```python
from build123d import *

# Parameters (mm, degrees)
BOSS_EXTRUDE1_DEPTH = 38.1
SHELL1_T            = -3.81
CUT_EXTRUDE1_DEPTH  = 3.81
BOSS_EXTRUDE2_DEPTH = 101.6
SKETCH5_W           = 24.13
SKETCH5_H           = 30.48
CUT_EXTRUDE2_DEPTH  = 97.79
BOSS_EXTRUDE3_DEPTH = 25.4


with BuildPart() as part:
    # Sketch1 → Boss-Extrude1 (new body)
    with BuildSketch(Plane.XY):
        Polygon((0, 0), (25.4, 0), (25.4, 5.08), (5.08, 101.6), (0, 101.6), align=None)
    extrude(amount=BOSS_EXTRUDE1_DEPTH)

    # Shell1
    shell1_openings = [part.faces().sort_by_distance(p)[0] for p in [
        (15.24, 53.34, 19.05),
    ]]
    offset(amount=SHELL1_T, openings=shell1_openings, kind=Kind.INTERSECTION)

    # Sketch2 → Cut-Extrude1 (cut)
    with BuildSketch(Plane.XZ):
        with BuildLine():
            Line((6.35, 22.225), (19.05, 22.225))
            ThreePointArc((19.05, 22.225), (22.225, 19.05), (19.05, 15.875))
            Line((19.05, 15.875), (6.35, 15.875))
            ThreePointArc((6.35, 15.875), (3.175, 19.05), (6.35, 22.225))
        make_face()
    extrude(amount=-CUT_EXTRUDE1_DEPTH, mode=Mode.SUBTRACT)

    # Sketch3 → Boss-Extrude2 (add)
    with BuildSketch(Plane(origin=(0, 101.6, 0), x_dir=(1, 0, 0), z_dir=(0, 1, 0))):
        Polygon((-19.05, 0), (0, -19.05), (0, 0), align=None)
        Polygon((0, -38.1), (0, -19.05), (-19.05, -38.1), align=None)
    extrude(amount=-BOSS_EXTRUDE2_DEPTH)

    # Sketch5 → Cut-Extrude2 (cut)
    with BuildSketch(Plane(origin=(0, 101.6, 0), x_dir=(1, 0, 0), z_dir=(0, 1, 0))):
        with Locations((13.335, -19.05)):
            Rectangle(SKETCH5_W, SKETCH5_H)
    extrude(amount=-CUT_EXTRUDE2_DEPTH, mode=Mode.SUBTRACT)

    # Sketch6 → Boss-Extrude3 (add)
    with BuildSketch(Plane.XZ):
        Polygon((-19.05, 0), (0, 19.05), (-19.05, 38.1), align=None)
    extrude(amount=-BOSS_EXTRUDE3_DEPTH)


solid = part.part
```
The listing builds one solid part. Answer for the finished solid, in the listing's coordinates (mm). A direction names the side the tool comes from. Round coordinates to 2 decimals unless told otherwise and drop trailing zeros. Order: outer loops, then holes, each group sorted by start corner. A loop starts at its lowest first (then second) coordinate and runs counter-clockwise, first axis right, second up. Notation, with made-up numbers: (-23, 2) - (2, 2) arc R22 cw to (2, 32) - close; hole circle Ø5 at (53.5, 4). An arc over 180 degrees is marked (long way). Put each result on its own line as item: value. Start each with the question number.
(1) Find section D-D (y = 69.5). Give the vertices of the cut face in (x, z), plus the area to 3 significant figures.
(2) Find section A-A (x = -2). Give the vertices of the cut face in (y, z).
(3) Find section B-B (z = 7.5). Give the vertices of the cut face in (x, y).
(4) Straight lines are drawn through the part: probe 1 along Z at (x, y) = (17, 13.5); probe 2 along Y at (x, z) = (17, 27); probe 3 along Z at (x, y) = (-9.5, 38). For each, find the intervals that lie inside material, in ascending order. Write a range as from..to.
(5) Given P1, Ø1.5, axis at x = 4.5, z = 28.5, coming from the -Y side; P2, Ø19.5, axis at x = 17.5, z = 19.5, coming from the +Y side; P3, Ø12, axis at y = 83.5, z = 25.5, coming from the +X side; P4, Ø6, axis at y = 87.5, z = 33.5, coming from the +X side, each flat-ended and moving along its own axis, determine where each tip first touches the part or whether it passes through.
(6) Determine the mould class of faces 6 (the cylindrical face through (22.224, 1.878, 19.12)), 7 (the flat face through (10, 43, 3.81)), 8 (the flat face through (-1, 52, 0)), 9 (the flat face through (25.4, 2, 19)) for opening direction Z: released by +Z, released by -Z, zero draft, split by the parting line, or undercut.
(7) Find section C-C (y = 82). Give the vertices of the cut face in (x, z).
(8) For faces 1 (the flat face through (15.382, 52.664, 1.878)), 2 (the flat face through (-9.66, 64.03, 9.39)), 3 (the flat face through (13, 2, 15.875)), 4 (the flat face through (10, 43, 34.29)), 5 (the flat face through (3, 0, 19)), determine the directions among +Z, -Z, +X, -X, +Y, -Y from which every point of the face is accessible in a straight line to the end or side of a thin tool.
Reply:
1. outline: (-19.05, 0) - (11.84, 0) - (11.84, 3.81) - (1.27, 3.81) - (1.27, 34.29) - (11.84, 34.29) - (11.84, 38.1) - (-19.05, 38.1) - (0, 19.05) - close
1. area: 492 mm^2
2. outline: (0, 0) - (101.6, 0) - (101.6, 17.05) - (25.4, 17.05) - (25.4, 21.05) - (101.6, 21.05) - (101.6, 38.1) - (0, 38.1) - close
3. outline: (-19.05, 0) - (25.4, 0) - (25.4, 3.81) - (1.27, 3.81) - (1.27, 101.6) - (-11.55, 101.6) - (-11.55, 25.4) - (-19.05, 25.4) - close
4. probe 1: 0..3.81, 34.29..38.1
4. probe 2: 0..3.81
4. probe 3: 0..9.55, 28.55..38.1
5. P1: y = 0
5. P2: y = 3.81
5. P3: x = 1.27
5. P4: x = 8.66
6. face 6: undercut
6. face 7: undercut
6. face 8: released by -Z
6. face 9: zero draft
7. outline: (-19.05, 0) - (9.21, 0) - (9.21, 3.81) - (1.27, 3.81) - (1.27, 34.29) - (9.21, 34.29) - (9.21, 38.1) - (-19.05, 38.1) - (0, 19.05) - close
8. face 1: +Z, -Z, +X, +Y
8. face 2: -X, +Y
8. face 3: +Y, -Y
8. face 4: +X, +Y
8. face 5: +Z, -Z, +X, -X, -Y
